Could you check a few things on this drawing? It's one solid part, dimensions in mm from its lowest x, y, z. Give positions to 0.01 mm unless a question says otherwise; leave off trailing zeros. Loops run counter-clockwise (first coordinate to the right, second up) from the corner with the lowest first, then second, coordinate; pieces in that order, holes last. Notation, with made-up numbers: M 10,88.5 L 61,88.5 A20 cw 61,108.5 Z; hole C 7,2.5 d10. An arc over 180 degrees is marked long. Write each question's results on one line, items separated by ' | '. Start each with the question number.
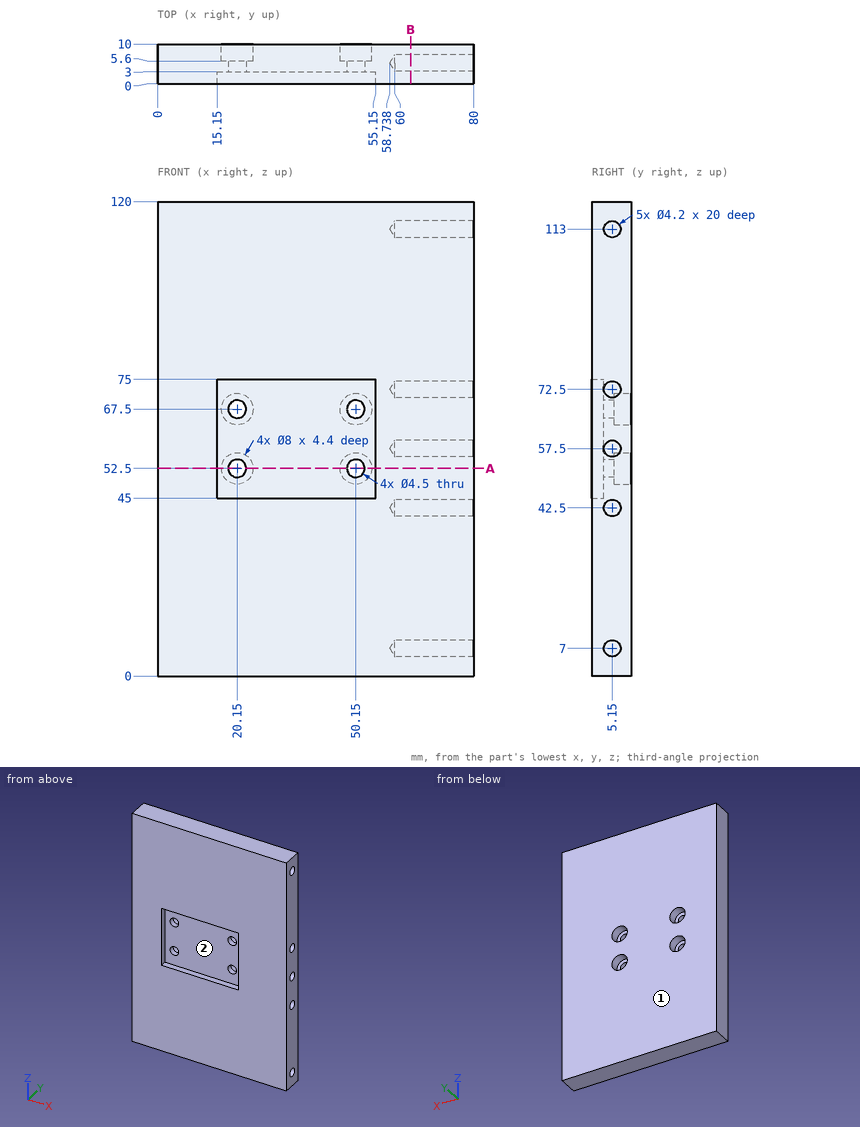
1) Thinking about a two-plate mould opening in Z: for the marked faces 1 and 2, which applies, pulls with the +Z half, pulls with the -Z half, needs draft (parallel to the pull), parting line crosses it, or undercut?
2) I'm going to push flat-ended pins straight in: P1, Ø6, axis at x = 20.15, z = 52.5, coming from the +Y side; P2, Ø9, axis at x = 50.15, z = 67.5, coming from the -Y side; P3, Ø3.5, axis at y = 5.15, z = 42.5, coming from the +X side; P4, Ø4, axis at x = 50.15, z = 67.5, coming from the +Y side. Where does each tip first touch, or does it pass through?
3) If we section it at A-A on z = 52.5: Write out the boundary of the cut face in (x, y), plus the area to 3 significant figures.
4) Please list where these lines run through material, in increasing order: line 1 (X direction, y = 9, z = 67.5); line 2 (Z direction, x = 64, y = 5) (1 decimal); line 3 (X direction, y = 4.5, z = 67.5). Write a range as from..to.
5) If we section it at B-B on x = 64: Write out the boundary of the cut face in (y, z), plus the area to 3 significant figures.
Calculated:
1) face 1: needs draft | face 2: undercut
2) P1: stops at y = 5.6 | P2: stops at y = 3 | P3: stops at x = 59.79 | P4: passes through
3) outline: M 0,0 L 15.15,0 L 15.15,3 L 17.9,3 L 17.9,5.6 L 16.15,5.6 L 16.15,10 L 0,10 Z; M 22.4,3 L 47.9,3 L 47.9,5.6 L 46.15,5.6 L 46.15,10 L 24.15,10 L 24.15,5.6 L 22.4,5.6 Z; M 52.4,3 L 55.15,3 L 55.15,0 L 80,0 L 80,10 L 54.15,10 L 54.15,5.6 L 52.4,5.6 Z | area: 586 mm2
4) line 1: x = 0..16.15, 24.15..46.15, 54.15..80 | line 2: z = 0..4.9, 9.1..40.4, 44.6..55.4, 59.6..70.4, 74.6..110.9, 115.1..120 | line 3: x = 0..17.9, 22.4..47.9, 52.4..80
5) outline: M 0,0 L 10,0 L 10,120 L 0,120 Z; hole C 5.15,7 d4.2; hole C 5.15,42.5 d4.2; hole C 5.15,57.5 d4.2; hole C 5.15,72.5 d4.2; hole C 5.15,113 d4.2 | area: 1,130 mm2
